Autodesk Inventor part; units mm, degrees
ref_plane "YZ Plane" through (0, 0, 0) normal (1, 0, 0) x (0, 1, 0)
ref_plane "XZ Plane" through (0, 0, 0) normal (0, 1, 0) x (-1, 0, 0)
ref_plane "XY Plane" through (0, 0, 0) normal (0, 0, 1) x (1, 0, 0)
sketch "Sketch1" plane through (0, 0, 0) normal (0, 0, 1) x (1, 0, 0)
  line L0 (0, 0) -> (20, 0)
  line L1 (20, 0) -> (20, 20)
  line L2 (20, 20) -> (0, 20)
  line L3 (0, 20) -> (0, 0)
  line L4 (0, 0) -> (20, 0)
  line L5 (20, 0) -> (20, -20)
  line L6 (20, -20) -> (0, -20)
  line L7 (0, -20) -> (0, 0)
  line L8 (20, 0) -> (40, 0)
  line L9 (40, 0) -> (40, -20)
  line L10 (40, -20) -> (20, -20)
  line L11 (20, -20) -> (20, 0)
  line L12 (0, -20) -> (-20, -20)
  line L13 (-20, -20) -> (-20, 0)
  line L14 (-20, 0) -> (0, 0)
  line L15 (0, 0) -> (0, -20)
  line L16 (0, -20) -> (20, -20)
  line L17 (20, -20) -> (20, -40)
  line L18 (20, -40) -> (0, -40)
  line L19 (0, -40) -> (0, -20)
  dimension "d0" = 20
  dimension "d1" = 20
  dimension "d2" = 20
  dimension "d3" = 20
  dimension "d4" = 20
  dimension "d5" = 20
  dimension "d6" = 20
  dimension "d7" = 20
  dimension "d8" = 20
  dimension "d9" = 20
extrude "Extrusion1" add sketch "Sketch1" along normal blind 3.8
sketch "Sketch2" plane through (0, 0, 3.8) normal (0, 0, 1) x (1, 0, 0)
  line L0 (-20, 0) -> (-20, -20)
  line L1 (-20, -8.2) -> (0, -8.2)
  line L2 (0, -8.2) -> (0, -11.8)
  line L3 (0, -11.8) -> (-20, -11.8)
  line L4 (-20, -11.8) -> (-20, -8.2)
  line L5 (-20, -20) -> (0, -20)
  line L6 (0, 0) -> (20, 0)
  line L7 (20, 0) -> (20, -20)
  line L8 (20, -20) -> (0, -20)
  line L9 (0, -20) -> (0, 0)
  line L10 (40, -20) -> (40, 0)
  line L11 (20, -8.2) -> (40, -8.2)
  line L12 (40, -8.2) -> (40, -11.8)
  line L13 (40, -11.8) -> (20, -11.8)
  line L14 (20, -11.8) -> (20, -8.2)
  line L15 (20, 20) -> (0, 20)
  line L16 (8.2, 0) -> (11.8, 0)
  line L17 (11.8, 0) -> (11.8, 20)
  line L18 (11.8, 20) -> (8.2, 20)
  line L19 (8.2, 20) -> (8.2, 0)
  line L20 (0, -40) -> (20, -40)
  line L21 (8.2, -20) -> (11.8, -20)
  line L22 (11.8, -20) -> (11.8, -40)
  line L23 (11.8, -40) -> (8.2, -40)
  line L24 (8.2, -40) -> (8.2, -20)
  dimension "d12" = 8.2
  dimension "d13" = 8.2
  dimension "d14" = 20
  dimension "d15" = 8.2
  dimension "d16" = 8.2
  dimension "d17" = 8.2
  dimension "d18" = 8.2
  dimension "d19" = 8.2
  dimension "d20" = 8.2
extrude "Extrusion2" add sketch "Sketch2" along normal blind 16.2 contours L1 L2 L3 L0 | L9 L6 L7 L8 L2 | L19 L15 L17 L6 | L8 L22 L20 L24 | L11 L10 L13 L7
sketch "Sketch3" plane through (0, 0, 20) normal (0, 0, 1) x (1, 0, 0)
  line L0 (0, 0) -> (0, -8.2)
  line L1 (0, 0) -> (0, -3.8)
  line L2 (0, -3.8) -> (8.2, -3.8)
  line L3 (8.2, -3.8) -> (8.2, -16.2)
  line L4 (8.2, -16.2) -> (0, -16.2)
  line L5 (0, -11.8) -> (0, -20)
  line L6 (0, -16.2) -> (0, -20)
  line L7 (20, -40) -> (20, -20)
  line L8 (0, -20) -> (20, -20)
  line L9 (20, -20) -> (20, -16.2)
  line L10 (20, -20) -> (20, -11.8)
  line L11 (20, -16.2) -> (11.8, -16.2)
  line L12 (11.8, -16.2) -> (11.8, -3.8)
  line L13 (11.8, -3.8) -> (20, -3.8)
  line L14 (20, -8.2) -> (20, 0)
  line L15 (8.2, 0) -> (0, 0)
  line L16 (20, 0) -> (0, 0)
  line L17 (40, 0) -> (20, 0)
  line L18 (20, 0) -> (20, -3.8)
  dimension "d23" = 3.8
  dimension "d24" = 8.2
  dimension "d25" = 12.4
  dimension "d26" = 8.2
extrude "Extrusion3" add sketch "Sketch3" along normal blind 19.8
sketch "Sketch4" plane through (11.8, 0, 3.8) normal (1, 0, 0) x (0, 0, -1)
  circle A0 centre (-8.2, 10) radius 2.25
  line L0 (-16.2, 0) -> (-16.2, 20)
  line L1 (0, 20) -> (-16.2, 20)
  point P0 (3.8, 0)
  dimension "d29" = 4.5
  dimension "d30" = 8
  dimension "d31" = 10
extrude "Extrusion4" cut sketch "Sketch4" against normal through all
sketch "Sketch5" plane through (11.8, -40, 3.8) normal (1, 0, 0) x (0, 0, -1)
  circle A0 centre (-8.2, 10) radius 2.25
  line L0 (-16.2, 0) -> (-16.2, 20)
  line L1 (0, 0) -> (-16.2, 0)
  point P0 (3.8, 40)
  dimension "d34" = 4.5
  dimension "d35" = 8
  dimension "d36" = 10
extrude "Extrusion5" cut sketch "Sketch5" against normal through all
sketch "Sketch6" plane through (11.8, -16.2, 20) normal (1, 0, 0) x (0, 0, -1)
  circle A0 centre (-10, 6.2) radius 2.25
  line L0 (0, 4.4) -> (0, 8)
  line L1 (16.2, 16.2) -> (-19.8, 16.2)
  point P0 (20, 16.2)
  dimension "d39" = 4.5
  dimension "d40" = 10
  dimension "d41" = 10
extrude "Extrusion6" cut sketch "Sketch6" against normal through all
sketch "Sketch7" plane through (20, -11.8, 3.8) normal (0, -1, 0) x (1, 0, 0)
  circle A0 centre (10, 8.2) radius 2.25
  line L0 (0, 16.2) -> (20, 16.2)
  line L1 (20, 0) -> (20, 16.2)
  point P0 (-20, -3.8)
  dimension "d44" = 4.5
  dimension "d45" = 8
  dimension "d46" = 10
extrude "Extrusion7" cut sketch "Sketch7" against normal through all
sketch "Sketch8" plane through (-20, -11.8, 3.8) normal (0, -1, 0) x (1, 0, 0)
  circle A0 centre (10, 8.2) radius 2.25
  line L0 (0, 16.2) -> (20, 16.2)
  line L1 (0, 0) -> (0, 16.2)
  point P0 (20, -3.8)
  dimension "d49" = 4.5
  dimension "d50" = 8
  dimension "d51" = 10
extrude "Extrusion8" cut sketch "Sketch8" against normal through all
fillet "Fillet1" radius 2 8 edges at (-10, 0, 0) (0, 10, 0) (-10, -20, 0) (0, -30, 0) (20, -30, 0) (30, -20, 0) (30, 0, 0) (20, 10, 0)
equation "\"d13\" = d12"
equation "\"d15\" = d12"
equation "\"d16\" = d12"
equation "\"d17\" = d12"
equation "\"d18\" = d12"
equation "\"d19\" = d12"
equation "\"d20\" = d12"
equation "\"d26\" = d24"
properties part number "fourwaylockver1"
Build history of the part. All positions in model axes, mm. A direction names the side the tool comes from. Coordinates: 2 decimals unless noted, no trailing zeros. Write each loop counter-clockwise with the first axis right and the second up, starting at its lowest first coordinate (ties: lowest second). Pieces come first, ordered by that corner, then holes.
1. Band-saw the part on C-C, the plane y = -10. Give the cut face in (x, z).
Answer block:
outline: (-20, 0) - (40, 0) - (40, 20) - (11.8, 20) - (11.8, 27.75) - (8.2, 27.75) - (8.2, 20) - (-20, 20) - close; (8.2, 32.25) - (11.8, 32.25) - (11.8, 39.8) - (8.2, 39.8) - close; hole circle Ø4.5 at (-10, 12); hole circle Ø4.5 at (30, 12)
2. Drop flat-ended pins along their axis: pin 1 (4 mm diameter, centred on y = -5, z = 18, fed in from -X); pin 2 (6 mm diameter, centred on y = -19, z = 8, fed in from +X); pin 3 (6 mm diameter, centred on y = 6, z = 25.5, fed in from -X); pin 4 (2 mm diameter, centred on y = 2, z = 10, fed in from -X). Give the stop position or say it passes through.
Answer block:
pin 1: stops at x = 0
pin 2: stops at x = 20
pin 3: passes through
pin 4: stops at x = 8.2
3. 3-axis set-ups, long thin cutter, end or side, ignore diameter. For faces 1 (the flat face through (16, -30, 3.8)), 2 (the flat face through (30, 0, 3)), 3 (the flat face through (30, -20, 3)): which of +Z, -Z, +X, -X, +Y, -Y reach the whole face in a straight line?
Answer block:
face 1: +Z, +X, -Y
face 2: +Z, -Z, +X, +Y
face 3: +Z, -Z, +X, -Y
4. Pull direction Y, two halves, no side cores. Call faces 4 (the flat face through (8.2, -9.9, 27.6)), 5 (the flat face through (10, 10, 20)), 6 (the flat face through (11.8, -10.1, 27.6)), 7 (the cylindrical face through (-9.15, -19.4, 0.57)): released by +Y, released by -Y, zero draft, split by the parting line, or undercut.
Answer block:
face 4: undercut
face 5: zero draft
face 6: undercut
face 7: released by -Y
5. Band-saw the part on D-D, the plane x = -10. Give the cut face in (y, z), and give its area (3 significant figures).
Answer block:
outline: (-20, 2) arc R2 ccw to (-18, 0) - (-2, 0) arc R2 ccw to (0, 2) - (0, 3.8) - (-8.2, 3.8) - (-8.2, 9.75) - (-11.8, 9.75) - (-11.8, 3.8) - (-20, 3.8) - close; (-11.8, 14.25) - (-8.2, 14.25) - (-8.2, 20) - (-11.8, 20) - close
area: 116 mm2
6. Drill centre lines: probe 1 along Y at (x, z) = (9.25, 12); probe 2 along Y at (x, z) = (8.5, 11); probe 3 along Y at (x, z) = (18, 6). Where is each one in solid material? Low to high.
Answer block:
probe 1: y = -40 to -32.25, -27.75 to 7.75, 12.25 to 20
probe 2: y = -40 to -32.02, -27.98 to 7.98, 12.02 to 20
probe 3: y = -20 to 0
7. Band-saw the part on B-B, the plane z = 30. Give the cut face in (x, y), and give its area (3 significant figures).
Answer block:
outline: (0, -20) - (20, -20) - (20, -16.2) - (11.8, -16.2) - (11.8, -12.25) - (8.2, -12.25) - (8.2, -16.2) - (0, -16.2) - close; (0, -3.8) - (8.2, -3.8) - (8.2, -7.75) - (11.8, -7.75) - (11.8, -3.8) - (20, -3.8) - (20, 0) - (0, 0) - close
area: 180 mm2
8. Band-saw the part on A-A, the plane y = -30. Give the cut face in (x, z), and give its area (3 significant figures).
Answer block:
outline: (0, 2) arc R2 ccw to (2, 0) - (18, 0) arc R2 ccw to (20, 2) - (20, 3.8) - (11.8, 3.8) - (11.8, 9.75) - (8.2, 9.75) - (8.2, 3.8) - (0, 3.8) - close; (8.2, 14.25) - (11.8, 14.25) - (11.8, 20) - (8.2, 20) - close
area: 116 mm2
